Drawing for the job (mm, zero at the part's lowest x, y, z). Coordinates: 2 decimals unless noted, no trailing zeros. Order: outer loops, then holes, each group sorted by start corner. A loop starts at its lowest first (then second) coordinate and runs counter-clockwise, first axis right, second up. Notation, with made-up numbers: M 47.5,58.5 L 51.5,58.5 A16 ccw 51.5,70.5 Z; hole C 83.25,-40 d11. An arc over 180 degrees is marked long. Write item = value, one per line. Start each with the question number.
Q1. Drill centre lines: probe 1 along Z at (x, y) = (28, 19); probe 2 along Z at (x, y) = (27, 9). Where is each one in solid material? Low to high.
Q2. Band-saw the part on A-A on y = 28. Write the cut outline in (x, z), plus the area to 3 significant figures.
Q3. Band-saw the part on B-B on x = 25.5. Write the cut outline in (y, z).
Q4. Pin check, flat tips, straight feed: P1, Ø8, axis at x = 36.5, y = 11, coming from the -Z side; P2, Ø8, axis at x = 35, y = 10.5, coming from the +Z side; P3, Ø12, axis at x = 13.5, y = 40, coming from the -Z side. Stop position of each tip, or through.
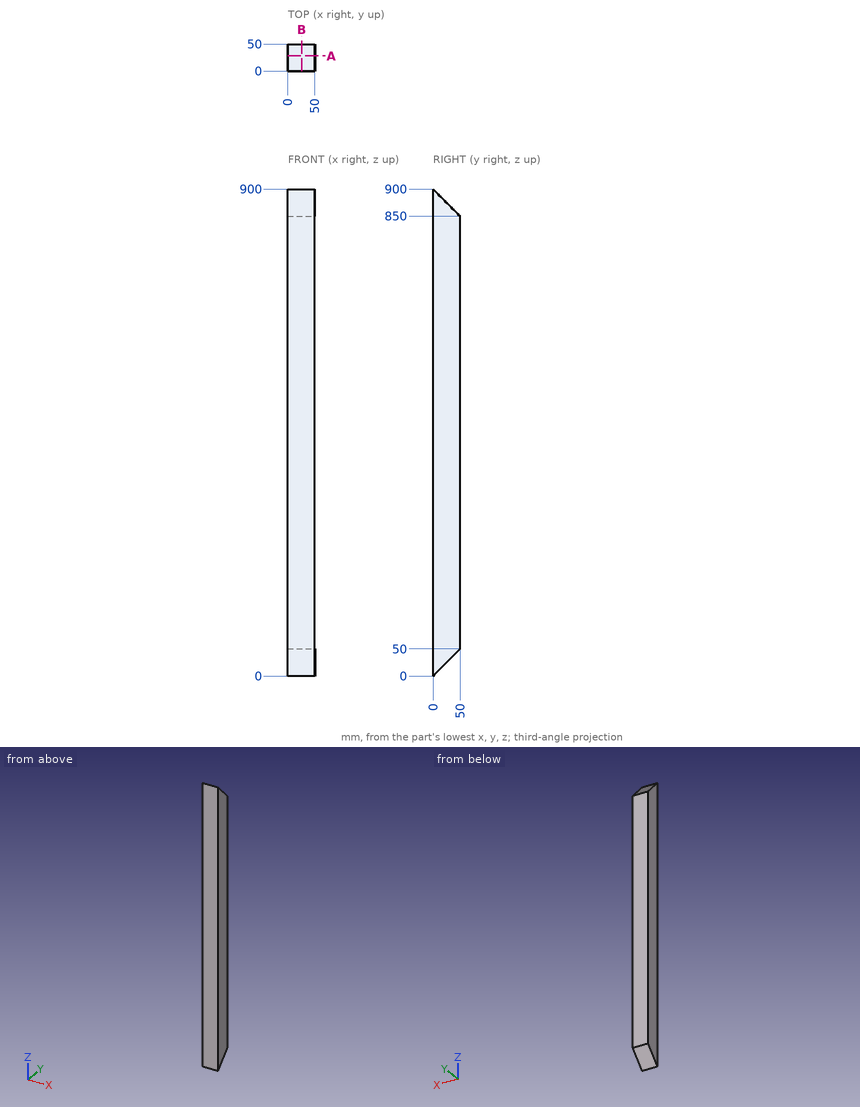
Recorded:
q1.probe_1 = 19 to 881
q1.probe_2 = 9 to 891
q2.outline = M 0,28 L 50,28 L 50,872 L 0,872 Z
q2.area = 42,200 mm2
q3.outline = M 0,0 L 50,50 L 50,850 L 0,900 Z
q4.P1 = 7
q4.P2 = 893.5
q4.P3 = 34
